```python
from build123d import *

# Parameters (mm, degrees)
SKETCH_1_W          = 60
SKETCH_1_H          = 80
EXTRUDE_1_DEPTH     = 3
SKETCH_2_R          = 11.5
SKETCH_2_R_2        = 1.75
SKETCH_2_R_3        = 4.25
CUT_EXTRUDE_1_DEPTH = 4
FILLET_1_R          = 2


with BuildPart() as part:
    # 草图1 → 凸台-拉伸1 (new body)
    with BuildSketch(Plane.XY):
        with Locations((30, 40)):
            Rectangle(SKETCH_1_W, SKETCH_1_H)
    extrude(amount=EXTRUDE_1_DEPTH)

    # 草图2 → 切除-拉伸1 (cut, through all)
    with BuildSketch(Plane.XY.offset(3)):
        with Locations((30, 21)):
            Circle(SKETCH_2_R)
        with Locations((19.393398282, 31.606601718)):
            Circle(SKETCH_2_R_2)
        with Locations((40.606601718, 31.606601718)):
            Circle(SKETCH_2_R_2)
        with Locations((40.606601718, 10.393398282)):
            Circle(SKETCH_2_R_2)
        with Locations((19.393398282, 10.393398282)):
            Circle(SKETCH_2_R_2)
        with Locations((15, 65)):
            Circle(SKETCH_2_R_3)
        with Locations((45, 65)):
            Circle(SKETCH_2_R_3)
    extrude(amount=-CUT_EXTRUDE_1_DEPTH, mode=Mode.SUBTRACT)

    # 圆角1
    fillet_1_edges = [part.edges().sort_by_distance(p)[0] for p in [
        (0, 80, 1.5),
        (60, 80, 1.5),
        (60, 0, 1.5),
        (0, 0, 1.5),
    ]]
    fillet(fillet_1_edges, radius=FILLET_1_R)


solid = part.part
```
Design review of the part built by this model. Coordinates are the model's own, in mm. Coordinates: 2 decimals unless noted, no trailing zeros. Order: outer loops, then holes, each group sorted by start corner. A loop starts at its lowest first (then second) coordinate and runs counter-clockwise, first axis right, second up.
1) Wall thickness on line 1 along Y through (x, z) = (45, 1.5); line 2 along Y through (x, z) = (30, 1.65); line 3 along Y through (x, z) = (39.5, 1.65): over which ranges is each line inside the solid? List them lowest first.
2) Take a section at B-B, the plane y = 65. Give the boundary of the cut face in (x, z), and give its area (3 significant figures).
3) Clearance check with a flat-ended pin moving along its axis: pin 1 (20.5 mm diameter, centred on x = 30, y = 21, fed in from +Z). State where the tip first meets the part, or that it passes through.
4) Take a section at D-D, the plane z = 0.85. Give the boundary of the cut face in (x, y), and give its area (3 significant figures).
5) Take a section at A-A, the plane x = 15. Give the boundary of the cut face in (y, z).
6) Take a section at C-C, the plane y = 21. Give the boundary of the cut face in (x, z), and give its area (3 significant figures).
7) Mouldability with a two-part tool opening along Y and no side actions: class faces 1 (the flat face through (30, 0, 1)), 2 (the flat face through (60, 39, 1)), 3 (the cylindrical face through (21.01, 30.94, 1.52)) as +Y half, -Y half, draft (parallel to the pull), parting line (faces both ways), or undercut.
Returned:
1. line 1: y = 0 to 60.75, 69.25 to 80
1. line 2: y = 0 to 9.5, 32.5 to 80
1. line 3: y = 0 to 9.04, 11.75 to 14.52, 27.48 to 30.25, 32.96 to 80
2. outline: (0, 0) - (10.75, 0) - (10.75, 3) - (0, 3) - close; (19.25, 0) - (40.75, 0) - (40.75, 3) - (19.25, 3) - close; (49.25, 0) - (60, 0) - (60, 3) - (49.25, 3) - close
2. area: 129 mm2
3. pin 1: passes through
4. outline: (0, 2) arc R2 ccw to (2, 0) - (58, 0) arc R2 ccw to (60, 2) - (60, 78) arc R2 ccw to (58, 80) - (2, 80) arc R2 ccw to (0, 78) - close; hole circle Ø8.5 at (15, 65); hole circle Ø3.5 at (19.39, 10.39); hole circle Ø3.5 at (19.39, 31.61); hole circle Ø23 at (30, 21); hole circle Ø3.5 at (40.61, 10.39); hole circle Ø3.5 at (40.61, 31.61); hole circle Ø8.5 at (45, 65)
4. area: 4,230 mm2
5. outline: (0, 0) - (60.75, 0) - (60.75, 3) - (0, 3) - close; (69.25, 0) - (80, 0) - (80, 3) - (69.25, 3) - close
6. outline: (0, 0) - (18.5, 0) - (18.5, 3) - (0, 3) - close; (41.5, 0) - (60, 0) - (60, 3) - (41.5, 3) - close
6. area: 111 mm2
7. face 1: -Y half
7. face 2: draft
7. face 3: undercut
